```python
from build123d import *

# Parameters (mm, degrees)
F3_DEPTH = 19.05
F2_R     = 9.525
F4_DEPTH = 25.4


with BuildPart() as f1:
    # F0 (on Front) → F1 (revolve)
    with BuildSketch(Plane.XZ):
        Polygon((-76.2, 0), (-6.35, 0), (-6.35, 38.1), (-12.7, 38.1), (-12.7, 50.8), (-25.4, 50.8), (-25.4, 19.05), (-63.5, 19.05), (-63.5, 76.2), (-76.2, 76.2), align=None)
    revolve(axis=Axis((0, 0, 38.1), (0, 0, 1)))

    # F2 (on Top) → F3 (join)
    with BuildSketch(Plane.XY):
        with BuildLine():
            Line((-107.95, -76.2), (0, -76.2))
            ThreePointArc((0, -76.2), (-53.8815367264, -53.8815367264), (-76.2, 0))
            Line((-76.2, 0), (-76.2, -38.1))
            Line((-76.2, -38.1), (-107.95, -38.1))
            Line((-107.95, -38.1), (-107.95, -47.625))
            ThreePointArc((-107.95, -47.625), (-101.2148079092, -50.4148079092), (-98.425, -57.15))
            ThreePointArc((-98.425, -57.15), (-101.2148079092, -63.8851920908), (-107.95, -66.675))
            Line((-107.95, -66.675), (-107.95, -76.2))
        make_face()
        with BuildLine():
            ThreePointArc((-107.95, -38.1), (-127, -57.15), (-107.95, -76.2))
            Line((-107.95, -76.2), (-107.95, -66.675))
            ThreePointArc((-107.95, -66.675), (-117.475, -57.15), (-107.95, -47.625))
            Line((-107.95, -47.625), (-107.95, -38.1))
        make_face()
    extrude(amount=F3_DEPTH)

    # F2 (on Top) → F4 (join)
    with BuildSketch(Plane.XY):
        with BuildLine():
            Line((107.95, -66.675), (107.95, -76.2))
            ThreePointArc((107.95, -76.2), (127, -57.15), (107.95, -38.1))
            Line((107.95, -38.1), (107.95, -47.625))
            ThreePointArc((107.95, -47.625), (114.6851920908, -50.4148079092), (117.475, -57.15))
            ThreePointArc((117.475, -57.15), (114.6851920908, -63.8851920908), (107.95, -66.675))
        make_face()
        with BuildLine():
            ThreePointArc((-76.2, 0), (-53.8815367264, -53.8815367264), (0, -76.2))
            Line((0, -76.2), (107.95, -76.2))
            Line((107.95, -76.2), (107.95, -66.675))
            ThreePointArc((107.95, -66.675), (98.425, -57.15), (107.95, -47.625))
            Line((107.95, -47.625), (107.95, -38.1))
            Line((107.95, -38.1), (76.2, -38.1))
            Line((76.2, -38.1), (76.2, 0))
            Line((76.2, 0), (76.2, 38.1))
            Line((76.2, 38.1), (107.95, 38.1))
            ThreePointArc((107.95, 38.1), (127, 57.15), (107.95, 76.2))
            Line((107.95, 76.2), (0, 76.2))
            Line((0, 76.2), (-107.95, 76.2))
            ThreePointArc((-107.95, 76.2), (-127, 57.15), (-107.95, 38.1))
            Line((-107.95, 38.1), (-76.2, 38.1))
            Line((-76.2, 38.1), (-76.2, 0))
        make_face()
        with Locations((-107.95, 57.15)):
            Circle(F2_R, mode=Mode.SUBTRACT)
        with Locations((107.95, 57.15)):
            Circle(F2_R, mode=Mode.SUBTRACT)
    extrude(amount=F4_DEPTH)


solid = f1.part
```
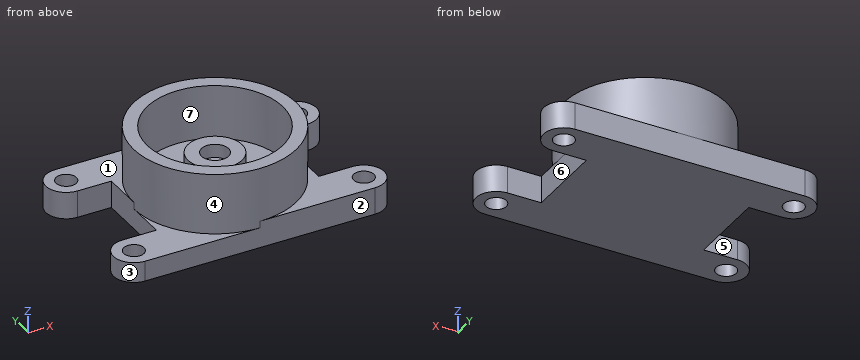
Verification items for the finished model (mm, model axes). Face numbers are marked on the shaded views. A direction names the side the tool comes from. Coordinates: 2 decimals unless noted, no trailing zeros. Write each loop counter-clockwise with the first axis right and the second up, starting at its lowest first coordinate (ties: lowest second). Pieces come first, ordered by that corner, then holes. Notation, with made-up numbers: M 19.25,37.5 L 78.25,37.5 A18 cw 78.25,43.5 Z; hole C -11.5,25 d10. An arc over 180 degrees is marked long. One line per item, written item: value.
Item 1: Mould release check, pull along Y, two halves, no side actions. Record for the marked faces 1, 2, 3 and 4: pulls with the +Y half, pulls with the -Y half, needs draft (parallel to the pull), parting line crosses it, or undercut.
Check sheet entries:
face 1: needs draft
face 2: pulls with the -Y half
face 3: undercut
face 4: parting line crosses it
Item 2: Section check A-A, the plane y = 57.15. Record the boundary of the cut face in (x, z) (3 decimals), plus the area to 3 significant figures.
Check sheet entries:
outline: M -127,0 L -117.475,0 L -117.475,25.4 L -127,25.4 Z; M -98.425,0 L 98.425,0 L 98.425,25.4 L 50.402,25.4 L 50.402,76.2 L 27.679,76.2 L 27.679,25.4 L -27.679,25.4 L -27.679,76.2 L -50.402,76.2 L -50.402,25.4 L -98.425,25.4 Z; M 117.475,0 L 127,0 L 127,25.4 L 117.475,25.4 Z
area: 7,790 mm^2
Item 3: Section check B-B, the plane z = 55. Record the boundary of the cut face in (x, y).
Check sheet entries:
outline: C 0,0 d152.4; hole C 0,0 d127
Item 4: Section check C-C, the plane y = 34.5. Record the boundary of the cut face in (x, z).
Check sheet entries:
outline: M -76.2,0 L 76.2,0 L 76.2,25.4 L 67.94,25.4 L 67.94,76.2 L 53.31,76.2 L 53.31,25.4 L -53.31,25.4 L -53.31,76.2 L -67.94,76.2 L -67.94,25.4 L -76.2,25.4 Z
Item 5: Gauge pin test, flat ends, axial feed: pin 1 Ø23 at (x, y) = (85, -47) entering from +Z; pin 2 Ø8 at (y, z) = (-3, 43) entering from -X; pin 3 Ø20.5 at (x, y) = (-5, 4) entering from +Z. Record the tip position at first contact, or that the pin passes through.
Check sheet entries:
pin 1: stops at z = 25.4
pin 2: stops at x = -76.2
pin 3: stops at z = 50.8
Item 6: Access from +Z, -Z, +X, -X, +Y, -Y to the whole of each face (thin tool, end or side, straight path). Record for the marked faces 5, 6 and 7.
Check sheet entries:
face 5: +Z, -Z, -X
face 6: +Z, -Z, +X
face 7: +Z
Item 7: Scan lines: line 1 along Y through (x, z) = (107.95, 18.75) (3 decimals); line 2 along X through (y, z) = (0, 47.75). Record each from-to range of solid material in increasing order.
Check sheet entries:
line 1: y = -76.2 to -66.675, -47.625 to -38.1, 38.1 to 47.625, 66.675 to 76.2
line 2: x = -76.2 to -63.5, -25.4 to -12.7, 12.7 to 25.4, 63.5 to 76.2
Item 8: Section check D-D, the plane y = -57.15. Record the boundary of the cut face in (x, z) (3 decimals).
Check sheet entries:
outline: M -127,0 L -117.475,0 L -117.475,19.05 L -127,19.05 Z; M -98.425,0 L 98.425,0 L 98.425,25.4 L 50.402,25.4 L 50.402,76.2 L 27.679,76.2 L 27.679,25.4 L -27.679,25.4 L -27.679,76.2 L -50.402,76.2 L -50.402,19.05 L -98.425,19.05 Z; M 117.475,0 L 127,0 L 127,25.4 L 117.475,25.4 Z
